```python
from build123d import *

# Parameters (mm, degrees)
SWEEP3_PROFILE_R    = 1.27
DOME1_FACE_RADIUS   = 1.27
DOME1_HEIGHT        = 0.889
SKETCH61_R          = 1.27
BOSS_EXTRUDE2_DEPTH = 30.48
SCALE1_SCALE        = 12.375


with BuildPart() as part:
    # Sweep3: sweep along a path in Sketch40
    with BuildLine(Plane.XY) as sweep3_path:
        Line((10.838928394, 0), (5.758928394, 0))
        ThreePointArc((5.758928394, 0), (3.472667092, 0.425853711), (1.49305551, 1.646296296))
        ThreePointArc((1.49305551, 1.646296296), (-2.217360492, -0.151058595), (1.702533775, -1.428595463))
    # Sweep3 profile (on start of the path) → Sweep3 (sweep)
    with BuildSketch(Plane(origin=(10.838928394, 0, 0), x_dir=(0, 0, -1), z_dir=(-1, 0, 0))):
        Circle(SWEEP3_PROFILE_R)
    sweep(path=sweep3_path.line)

    # Dome1: a dome of height H over a round flat face of radius A is a cap of a sphere of radius (A * A + H * H) / (2 * H)
    dome1_r = (DOME1_FACE_RADIUS * DOME1_FACE_RADIUS + DOME1_HEIGHT * DOME1_HEIGHT) / (2 * DOME1_HEIGHT)
    dome1_base = Plane((1.702533775, -1.428595463, 0), z_dir=(0.642787609687, 0.766044443119, 0))
    with Locations(dome1_base.offset(DOME1_HEIGHT - dome1_r)):
        dome1_ball = Sphere(dome1_r, mode=Mode.PRIVATE)
    add(split(dome1_ball, bisect_by=dome1_base, keep=Keep.TOP, mode=Mode.PRIVATE))

    # Sketch61 → Boss-Extrude2 (add)
    with BuildSketch(Plane(origin=(10.838928394, 0, 0), x_dir=(0, 0, -1), z_dir=(1, 0, 0))):
        Circle(SKETCH61_R)
    extrude(amount=BOSS_EXTRUDE2_DEPTH)


with BuildPart() as part_1:
    # Scale1: scaled about (16.50671912, 0.023905417, 0)
    add(part.part.scale(SCALE1_SCALE).moved(Location((-187.76392999, -0.271924118, 0))))


solid = part_1.part
```
Source: CAD feature listing. Evaluate the final solid. Frame: model axes, mm. Give positions to 0.01 mm unless a question says otherwise; leave off trailing zeros. Order: outer loops, then holes, each group sorted by start corner. A loop starts at its lowest first (then second) coordinate and runs counter-clockwise, first axis right, second up. Notation, with made-up numbers: (76.25, 61) -> (133.25, 61) arc R15 cw to (133.25, 69) -> close; hole circle Ø3 at (35, -38.5). An arc over 180 degrees is marked (long way). Use a Markdown table: item, result.
Q1. Material intervals for line 1 (Y direction, x = -195.5, z = 6); line 2 (Z direction, x = 202.5, y = 7); line 3 (Y direction, x = 188, z = 0.5), sorted ascending. Write a range as [from, to].
A:
| item | result |
|---|---|
| line 1 | [-41.58, -10.69], [10.15, 41.04] |
| line 2 | [-13.93, 13.93] |
| line 3 | [-15.98, 15.44] |
Q2. First-contact query: P1, Ø1, axis at x = 118.5, y = 17, coming from the -Z side; P2, Ø4, axis at x = 150.5, z = -12, coming from the +Y side; P3, Ø10, axis at y = 7, z = 0, coming from the -X side; P4, Ø6, axis at x = 77.5, z = 0.5, coming from the -Y side. Flat tips, straight axial feed; report the tip coordinate or a pass-through.
A:
| item | result |
|---|---|
| P1 | through |
| P2 | y = 11.85 |
| P3 | x = -230.92 |
| P4 | y = -15.99 |
Q3. Section B-B (x = -10). Return the cut outline in (y, z).
A:
| item | result |
|---|---|
| outline | circle Ø31.43 at (-0.27, 0) |
Q4. Section A-A (z = -10). Return the cut outline in (x, y).
A:
| item | result |
|---|---|
| outline | (-177.43, 11.12) arc R90.71 ccw to (-116.5, -12.4) -> (323.56, -12.4) -> (323.56, 11.85) -> (-116.5, 11.85) arc R66.46 cw to (-161.14, 29.08) arc R39.63 ccw (long way) to (-157.41, -25.74) arc R13.41 ccw to (-175.98, -10.16) arc R15.38 cw (long way) to start |
